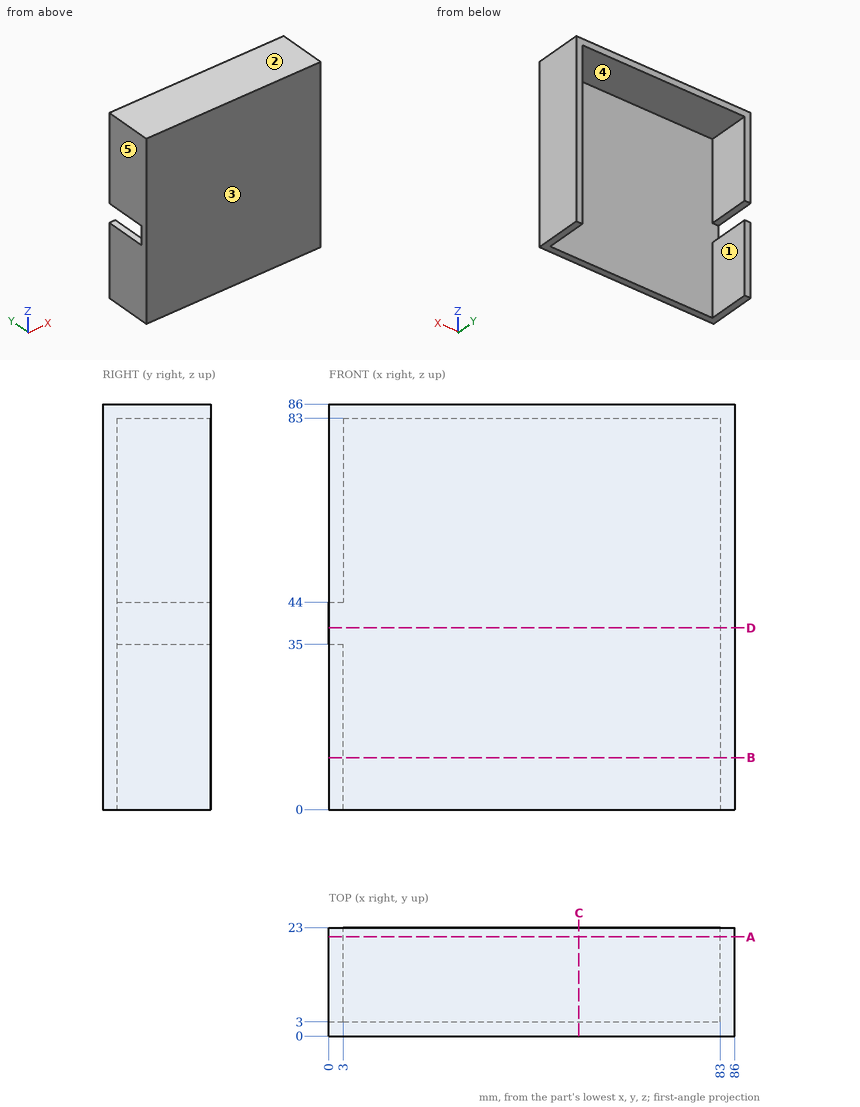
Source: three-view drawing plus pictorial views. Frame: mm from the lowest corner of the part. A direction names the side the tool comes from. Give positions to 0.01 mm unless a question says otherwise; leave off trailing zeros. Write each loop counter-clockwise with the first axis right and the second up, starting at its lowest first coordinate (ties: lowest second). Pieces come first, ordered by that corner, then holes.
(1) Ray query, line 1 (X direction, y = 12.5, z = 82); line 2 (Y direction, x = 33.5, z = 12.5); line 3 (Z direction, x = 16, y = 7.75). Return the intervals inside material, ascending.
(2) Cut plane A-A, the plane y = 21. Return loops of the section in (x, z).
(3) Mould query, pull axis X, two halves, no side actions, for the marked faces 3, 4 and 5. Classes: released by +X, released by -X, zero draft, split by the parting line, or undercut.
(4) Cut plane C-C, the plane x = 53. Return loops of the section in (y, z), then the cut area to 3 significant figures.
(5) Cut plane B-B, the plane z = 11. Return loops of the section in (x, y), then the cut area to 3 significant figures.
(6) Cut plane D-D, the plane z = 38.5. Return loops of the section in (x, y).
(7) Access query for the marked faces 1 and 2. Directions: +Z, -Z, +X, -X, +Y, -Y. A direction counts if a zero-diameter tool reaches every point of the face in a straight line with its end or side. Return the directions, or none.
(8) First-contact query: P1, Ø1.5, axis at x = 27.5, z = 65, coming from the +Y side; P2, Ø6, axis at x = 38.5, y = 14, coming from the -Z side. Flat tips, straight axial feed; report the tip coordinate or a pass-through.
Values follow:
1. line 1: x = 0 to 3, 83 to 86
1. line 2: y = 0 to 3
1. line 3: z = 83 to 86
2. outline: (0, 0) - (3, 0) - (3, 35) - (0, 35) - close; (0, 44) - (3, 44) - (3, 83) - (83, 83) - (83, 0) - (86, 0) - (86, 86) - (0, 86) - close
3. face 3: zero draft
3. face 4: undercut
3. face 5: released by -X
4. outline: (0, 0) - (3, 0) - (3, 83) - (23, 83) - (23, 86) - (0, 86) - close
4. area: 318 mm2
5. outline: (0, 0) - (86, 0) - (86, 23) - (83, 23) - (83, 3) - (3, 3) - (3, 23) - (0, 23) - close
5. area: 378 mm2
6. outline: (0, 0) - (86, 0) - (86, 23) - (83, 23) - (83, 3) - (0, 3) - close
7. face 1: -Z, +Y
7. face 2: +Z, +X, -X, +Y, -Y
8. P1: stops at y = 3
8. P2: stops at z = 83
